Model file for the job. Use its own axes, mm. Face numbers are marked on the shaded views. A direction names the side the tool comes from. Round coordinates to 2 decimals unless told otherwise and drop trailing zeros. Order: outer loops, then holes, each group sorted by start corner. A loop starts at its lowest first (then second) coordinate and runs counter-clockwise, first axis right, second up. Notation, with made-up numbers: (-35, 67.25) - (22, 67.25) arc R16 cw to (22, 88.25) - close; hole circle Ø3 at (8.25, 4.25). An arc over 180 degrees is marked (long way). Write item = value, one per line. Start each with the question number.
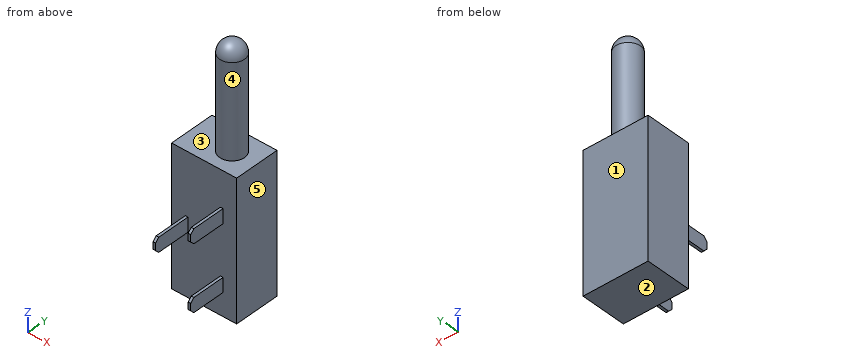
from build123d import *

# Parameters (mm, degrees)
SKETCH1_W           = 12.7
SKETCH1_H           = 8.89
BOSS_EXTRUDE1_DEPTH = 26.924
SKETCH2_R           = 2.4257
BOSS_EXTRUDE2_DEPTH = 20.574
FILLET1_R           = 2.4257
SKETCH3_W           = 0.508
SKETCH3_H           = 2.794
BOSS_EXTRUDE3_DEPTH = 7.112
CHAMFER1_SIZE       = 0.6985


with BuildPart() as part:
    # Sketch1 → Boss-Extrude1 (new body)
    with BuildSketch(Plane.XY):
        with Locations((-1.524, 0)):
            Rectangle(SKETCH1_W, SKETCH1_H)
    extrude(amount=-BOSS_EXTRUDE1_DEPTH)

    # Sketch2 → Boss-Extrude2 (add)
    with BuildSketch(Plane.XY):
        Circle(SKETCH2_R)
    extrude(amount=BOSS_EXTRUDE2_DEPTH)

    # Fillet1
    fillet1_edges = [part.edges().sort_by_distance(p)[0] for p in [
        (-2.4257, 0, 20.574),
    ]]
    fillet(fillet1_edges, radius=FILLET1_R)

    # Sketch3 → Boss-Extrude3 (add)
    with BuildSketch(Plane.XZ.offset(4.445)):
        with Locations((-4.953, -13.462)):
            Rectangle(SKETCH3_W, SKETCH3_H)
        with Locations((1.905, -21.082)):
            Rectangle(SKETCH3_W, SKETCH3_H)
        with Locations((1.905, -8.382)):
            Rectangle(SKETCH3_W, SKETCH3_H)
    extrude(amount=BOSS_EXTRUDE3_DEPTH)

    # Chamfer1
    chamfer1_edges = [part.edges().sort_by_distance(p)[0] for p in [
        (-4.953, -11.557, -14.859),
        (-4.953, -11.557, -12.065),
        (1.905, -11.557, -19.685),
        (1.905, -11.557, -22.479),
        (1.905, -11.557, -9.779),
        (1.905, -11.557, -6.985),
    ]]
    chamfer(chamfer1_edges, length=CHAMFER1_SIZE)


solid = part.part
Item 1: Saw through at B-B, the plane x = 0. Give the cut face in (y, z) (3 decimals).
Item 2: Saw through at A-A, the plane y = -9.5. Give the cut face in (x, z) (3 decimals), then the cut area to 3 significant figures.
Item 3: Drop flat-ended pins along their axis: pin 1 (2 mm diameter, centred on y = -8, z = -21, fed in from +X); pin 2 (5 mm diameter, centred on x = 2.5, y = -3.5, fed in from +Z); pin 3 (1.4 mm diameter, centred on y = -7, z = -13.5, fed in from +X). Give the stop position or say it passes through.
Item 4: Saw through at C-C, the plane y = 0. Give the cut face in (x, z), then the cut area to 3 significant figures.
Item 5: Saw through at D-D, the plane z = -11.5. Give the cut face in (x, y) (3 decimals).
Item 6: Probe L1, parallel to Y at x = -5.5, z = -6 (3 decimals); L2, parallel to Z at x = -4.5, y = -1; L3, parallel to Z at x = -5, y = -7.75 (3 decimals). List the from-to ranges inside material, lowest first.
Item 7: Which spindle directions (+Z, -Z, +X, -X, +Y, -Y) get a long thin tool onto all of the face, cutting with end or side? Do the marked faces 4 and 5. Say none if no direction does.
Item 8: Mould opens along Z. For the marked faces 1, 2 and 3 say: +Z half, -Z half, draft (parallel to the pull), parting line (faces both ways), or undercut.
Check sheet entries:
q1.outline = (-4.445, -26.924) - (4.445, -26.924) - (4.445, 0) - (2.426, 0) - (2.426, 18.148) arc R2.426 ccw to (-2.426, 18.148) - (-2.426, 0) - (-4.445, 0) - close
q2.outline = (-5.207, -14.859) - (-4.699, -14.859) - (-4.699, -12.065) - (-5.207, -12.065) - close; (1.651, -22.479) - (2.159, -22.479) - (2.159, -19.685) - (1.651, -19.685) - close; (1.651, -9.779) - (2.159, -9.779) - (2.159, -6.985) - (1.651, -6.985) - close
q2.area = 4.26 mm2
q3.pin_1 = 2.16
q3.pin_2 = 19.77
q3.pin_3 = -4.7
q4.outline = (-7.87, -26.92) - (4.83, -26.92) - (4.83, 0) - (2.43, 0) - (2.43, 18.15) arc R2.43 ccw to (-2.43, 18.15) - (-2.43, 0) - (-7.87, 0) - close
q4.area = 439 mm2
q5.outline = (-7.874, -4.445) - (4.826, -4.445) - (4.826, 4.445) - (-7.874, 4.445) - close
q6.L1 = -4.445 to 4.445
q6.L2 = -26.92 to 0
q6.L3 = -14.859 to -12.065
q7.face_4 = +Z
q7.face_5 = +Z, -Z, +X, +Y, -Y
q8.face_1 = draft
q8.face_2 = -Z half
q8.face_3 = +Z half
